The model under review builds one solid part; all positions refer to its coordinate system, in mm. Face numbers are marked on the shaded views. A direction names the side the tool comes from. Coordinates: 2 decimals unless noted, no trailing zeros. Order: outer loops, then holes, each group sorted by start corner. A loop starts at its lowest first (then second) coordinate and runs counter-clockwise, first axis right, second up.
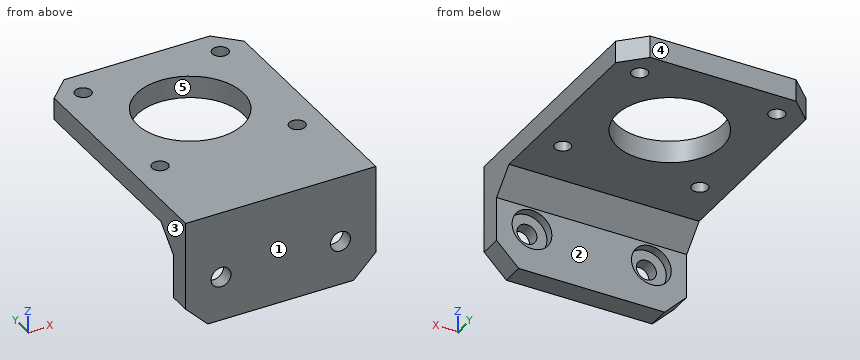
```python
from build123d import *

# Parameters (mm, degrees)
F0_W          = 43
F0_H          = 43
F0_R          = 1.8
F0_R_2        = 12
F0_H_2        = 10
F1_DEPTH      = 5
F0_H_3        = 5
F2_DEPTH      = 5
F2_DEPTH_BACK = 20
F3_R          = 2.25
F4_DEPTH      = 5
F3_R_2        = 4.5
F5_DEPTH      = 2
F6_SIZE       = 5


with BuildPart() as f1:
    # F0 (on Top) → F1 (new body)
    with BuildSketch(Plane.XY):
        Rectangle(F0_W, F0_H)
        with Locations((-15.5, -15.5)):
            Circle(F0_R, mode=Mode.SUBTRACT)
        with Locations((15.5, -15.5)):
            Circle(F0_R, mode=Mode.SUBTRACT)
        with Locations((-15.5, 15.5)):
            Circle(F0_R, mode=Mode.SUBTRACT)
        Circle(F0_R_2, mode=Mode.SUBTRACT)
        with Locations((15.5, 15.5)):
            Circle(F0_R, mode=Mode.SUBTRACT)
        with Locations((0, -26.5)):
            Rectangle(F0_W, F0_H_2)
    extrude(amount=F1_DEPTH)

    # F0 (on Top) → F2 (join, two sides)
    with BuildSketch(Plane.XY) as f2_sk:
        with Locations((0, -34)):
            Rectangle(F0_W, F0_H_3)
    extrude(amount=F2_DEPTH)
    extrude(f2_sk.sketch, amount=-F2_DEPTH_BACK)

    # F3 (on face) → F4 (cut, through all)
    with BuildSketch(Plane(origin=(0, -31.5, 0), x_dir=(-1, 0, 0), z_dir=(0, 1, 0))):
        with Locations((-13.5, -10)):
            Circle(F3_R)
        with Locations((13.5, -10)):
            Circle(F3_R)
    extrude(amount=-F4_DEPTH, mode=Mode.SUBTRACT)

    # F3 (on face) → F5 (cut)
    with BuildSketch(Plane(origin=(0, -31.5, 0), x_dir=(-1, 0, 0), z_dir=(0, 1, 0))):
        with Locations((-13.5, -10)):
            Circle(F3_R_2)
        with Locations((-13.5, -10)):
            Circle(F3_R, mode=Mode.SUBTRACT)
        with Locations((13.5, -10)):
            Circle(F3_R_2)
        with Locations((13.5, -10)):
            Circle(F3_R, mode=Mode.SUBTRACT)
    extrude(amount=-F5_DEPTH, mode=Mode.SUBTRACT)

    # F6
    f6_edges = [f1.edges().sort_by_distance(p)[0] for p in [
        (-21.5, 21.5, 2.5),
        (21.5, 21.5, 2.5),
        (-21.5, -34, -20),
        (21.5, -34, -20),
        (0, -31.5, 0),
    ]]
    chamfer(f6_edges, length=F6_SIZE)


solid = f1.part
```
(1) Draft analysis for pull direction Y (two halves, no side actions). For the marked faces 3, 4 and 5, state which applies: released by +Y, released by -Y, zero draft, split by the parting line, or undercut.
A:
face 3: zero draft
face 4: released by +Y
face 5: undercut
(2) Machinability: for the marked faces 1 and 2, which of the approach directions +Z, -Z, +X, -X, +Y, -Y give a long, thin tool a straight path to every point of the face, cutting with its end or side? Answer none if there is none.
A:
face 1: +Z, -Z, +X, -X, -Y
face 2: -Z, +X, -X, +Y
(3) We need section C-C, the plane y = 0. Write out the cut boundary in (x, z), and give its area (3 significant figures).
A:
outline: (-21.5, 0) - (-12, 0) - (-12, 5) - (-21.5, 5) - close; (12, 0) - (21.5, 0) - (21.5, 5) - (12, 5) - close
area: 95.0 mm2
(4) Wall thickness on probe 1 along Y at (x, z) = (0, 2.1); probe 2 along Y at (x, z) = (-15.5, 2.5); probe 3 along Y at (x, z) = (-19, -7.25): over which ranges is each line inside the solid? List them lowest first.
A:
probe 1: y = -36.5 to -12, 12 to 21.5
probe 2: y = -36.5 to -17.3, -13.7 to 13.7, 17.3 to 21.5
probe 3: y = -36.5 to -31.5
(5) We need section A-A, the plane x = 0. Write out the cut boundary in (y, z), and give its area (4 significant figures).
A:
outline: (-36.5, -20) - (-31.5, -20) - (-31.5, -5) - (-26.5, 0) - (-12, 0) - (-12, 5) - (-36.5, 5) - close; (12, 0) - (21.5, 0) - (21.5, 5) - (12, 5) - close
area: 282.5 mm2
(6) For pin 1 Ø5 at (x, z) = (-13.5, -10) entering from +Y; pin 2 Ø13 at (x, y) = (-1.5, -7.5) entering from -Z; pin 3 Ø11.5 at (x, z) = (13.5, -10) entering from +Y, all flat-tipped, find the tip position at first contact; note any pin that passes through.
A:
pin 1: stops at y = -33.5
pin 2: stops at z = 0
pin 3: stops at y = -30.75
(7) We need section D-D, the plane y = 15.5. Write out the cut boundary in (x, z), and give its area (3 significant figures).
A:
outline: (-21.5, 0) - (-17.3, 0) - (-17.3, 5) - (-21.5, 5) - close; (-13.7, 0) - (13.7, 0) - (13.7, 5) - (-13.7, 5) - close; (17.3, 0) - (21.5, 0) - (21.5, 5) - (17.3, 5) - close
area: 179 mm2
(8) We need section B-B, the plane z = -10. Write out the cut boundary in (x, y).
A:
outline: (-21.5, -36.5) - (-15.75, -36.5) - (-15.75, -33.5) - (-18, -33.5) - (-18, -31.5) - (-21.5, -31.5) - close; (-11.25, -36.5) - (11.25, -36.5) - (11.25, -33.5) - (9, -33.5) - (9, -31.5) - (-9, -31.5) - (-9, -33.5) - (-11.25, -33.5) - close; (15.75, -36.5) - (21.5, -36.5) - (21.5, -31.5) - (18, -31.5) - (18, -33.5) - (15.75, -33.5) - close
